Build history of the part. All positions in model axes, mm. A direction names the side the tool comes from. Coordinates: 2 decimals unless noted, no trailing zeros. Order: outer loops, then holes, each group sorted by start corner. A loop starts at its lowest first (then second) coordinate and runs counter-clockwise, first axis right, second up. Notation, with made-up numbers: (83, 56.25) -> (128, 56.25) arc R32 ccw to (128, 92.25) -> close; hole circle Ø9 at (-27.75, -18.75). An arc over 180 degrees is marked (long way). Write each question's results on one line, items separated by ' | '.
from build123d import *

# Parameters (mm, degrees)
SKETCH1_W           = 13
SKETCH1_H           = 30
BOSS_EXTRUDE1_DEPTH = 14
SKETCH2_W           = 13
SKETCH2_H           = 7
BOSS_EXTRUDE2_DEPTH = 18.33
SKETCH3_W           = 10
SKETCH3_H           = 14
CUT_EXTRUDE1_DEPTH  = 5.5
SKETCH4_W           = 14
SKETCH4_H           = 4
CUT_EXTRUDE2_DEPTH  = 46.224207014
FILLET1_R           = 3
CUT_EXTRUDE3_DEPTH  = 46.980744883
SKETCH6_W           = 7.5
SKETCH6_H           = 5.1
CUT_EXTRUDE4_DEPTH  = 39.771495973


with BuildPart() as part:
    # Sketch1 → Boss-Extrude1 (new body)
    with BuildSketch(Plane.XY):
        with Locations((6.5, 15)):
            Rectangle(SKETCH1_W, SKETCH1_H)
    extrude(amount=BOSS_EXTRUDE1_DEPTH)

    # Sketch2 → Boss-Extrude2 (add)
    with BuildSketch(Plane.XY.offset(14)):
        with Locations((6.5, 15)):
            Rectangle(SKETCH2_W, SKETCH2_H)
    extrude(amount=BOSS_EXTRUDE2_DEPTH)

    # Sketch3 → Cut-Extrude1 (cut)
    with BuildSketch(Plane(origin=(0, 18.5, 0), x_dir=(1, 0, 0), z_dir=(0, 1, 0))):
        with Locations((8, -22.33)):
            Rectangle(SKETCH3_W, SKETCH3_H)
    extrude(amount=-CUT_EXTRUDE1_DEPTH, mode=Mode.SUBTRACT)

    # Sketch4 → Cut-Extrude2 (cut, through all)
    with BuildSketch(Plane(origin=(3, 0, 0), x_dir=(0, 0, -1), z_dir=(1, 0, 0))):
        with Locations((-22.33, 15)):
            Rectangle(SKETCH4_W, SKETCH4_H)
    extrude(amount=-CUT_EXTRUDE2_DEPTH, mode=Mode.SUBTRACT)

    # Fillet1
    fillet1_edges = [part.edges().sort_by_distance(p)[0] for p in [
        (6.5, 11.5, 14),
        (6.5, 18.5, 14),
    ]]
    fillet(fillet1_edges, radius=FILLET1_R)

    # Sketch5 → Cut-Extrude3 (cut, through all)
    with BuildSketch(Plane.ZY):
        with BuildLine():
            Line((5.2, 5), (5.2, 11))
            ThreePointArc((5.2, 11), (7, 12.8), (8.8, 11))
            Line((8.8, 11), (8.8, 5))
            ThreePointArc((8.8, 5), (7, 3.2), (5.2, 5))
        make_face()
        with BuildLine():
            Line((5.2, 19), (5.2, 25))
            ThreePointArc((5.2, 25), (7, 26.8), (8.8, 25))
            Line((8.8, 25), (8.8, 19))
            ThreePointArc((8.8, 19), (7, 17.2), (5.2, 19))
        make_face()
    extrude(amount=-CUT_EXTRUDE3_DEPTH, mode=Mode.SUBTRACT)

    # Sketch6 → Cut-Extrude4 (cut, through all)
    with BuildSketch(Plane(origin=(0, 13, 0), x_dir=(1, 0, 0), z_dir=(0, 1, 0))):
        with Locations((9.25, -22.33)):
            Rectangle(SKETCH6_W, SKETCH6_H)
    extrude(amount=-CUT_EXTRUDE4_DEPTH, mode=Mode.SUBTRACT)


solid = part.part
Item 1: Pin check, flat tips, straight feed: pin 1 (1.5 mm diameter, centred on x = 7.5, z = 23.5, fed in from +Y); pin 2 (0.6 mm diameter, centred on y = 18, z = 20.5, fed in from +X); pin 3 (0.8 mm diameter, centred on y = 12.5, z = 22.5, fed in from +X); pin 4 (1.5 mm diameter, centred on x = 2, z = 22, fed in from -Y). Stop position of each tip, or through.
Answer:
pin 1: passes through | pin 2: stops at x = 3 | pin 3: stops at x = 5.5 | pin 4: stops at y = 11.5
Item 2: Pull direction Y, two halves, no side cores. Call faces 6 (the cylindrical face through (6.591, 19.752, 14.562)), 7 (the flat face through (6, 8, 8.8)), 8 (the flat face through (5, 11.5, 25)): released by +Y, released by -Y, zero draft, split by the parting line, or undercut.
Answer:
face 6: released by +Y | face 7: undercut | face 8: released by -Y
Item 3: Slice it at A-A, the plane y = 7.5. List the corners of the cut face in (x, z).
Answer:
outline: (0, 0) -> (13, 0) -> (13, 5.2) -> (0, 5.2) -> close; (0, 8.8) -> (13, 8.8) -> (13, 14) -> (0, 14) -> close
Item 4: Slice it at C-C, the plane x = 4.25. List the corners of the cut face in (y, z), and give its area (3 significant figures).
Answer:
outline: (0, 0) -> (30, 0) -> (30, 14) -> (21.5, 14) arc R3 cw to (19.01, 15.33) -> (13, 15.33) -> (13, 29.33) -> (18.5, 29.33) -> (18.5, 32.33) -> (11.5, 32.33) -> (11.5, 17) arc R3 cw to (8.5, 14) -> (0, 14) -> close; hole (5, 5.2) -> (11, 5.2) arc R1.8 ccw to (11, 8.8) -> (5, 8.8) arc R1.8 ccw to start; hole (19, 5.2) -> (25, 5.2) arc R1.8 ccw to (25, 8.8) -> (19, 8.8) arc R1.8 ccw to start | area: 411 mm^2
Item 5: Drill centre lines: line 1 (Z direction, x = 2, y = 23.75); line 2 (Y direction, x = 2.75, z = 5.5); line 3 (Z direction, x = 0.75, y = 12.5). Where is each one in solid material? Low to high. Write a range as from..to.
Answer:
line 1: z = 0..5.2, 8.8..14 | line 2: y = 0..4.01, 11.99..18.01, 25.99..30 | line 3: z = 0..6.01, 7.99..32.33
Item 6: Tool access for faces 1 (the flat face through (5.5, 12, 22)), 2 (the flat face through (6, 4, 14)), 3 (the flat face through (7, 16, 15.33)), 4 (the flat face through (6, 8, 5.2)), 5 (the flat face through (3, 18, 22)): list every direction of +Z, -Z, +X, -X, +Y, -Y with a clear straight run to the whole face (end or side of a thin tool).
Answer:
face 1: +X, +Y, -Y | face 2: +Z, +X, -X, -Y | face 3: +X | face 4: +X, -X | face 5: +X, +Y
Item 7: Slice it at D-D, the plane z = 7. List the corners of the cut face in (x, y).
Answer:
outline: (0, 0) -> (13, 0) -> (13, 3.2) -> (0, 3.2) -> close; (0, 12.8) -> (13, 12.8) -> (13, 17.2) -> (0, 17.2) -> close; (0, 26.8) -> (13, 26.8) -> (13, 30) -> (0, 30) -> close
Item 8: Slice it at B-B, the plane z = 21. List the corners of the cut face in (x, y), and give its area (4 significant figures).
Answer:
outline: (0, 11.5) -> (5.5, 11.5) -> (5.5, 13) -> (0, 13) -> close; (0, 17) -> (3, 17) -> (3, 18.5) -> (0, 18.5) -> close | area: 12.75 mm^2
